```python
from build123d import *

# Parameters (mm, degrees)
EXTRUDE_1_DEPTH              = 5
SKETCH_2_R                   = 6.25
EXTRUDE_2_DEPTH              = 3
SKETCH_3_R                   = 5
EXTRUDE_3_DEPTH              = 5
HOLE_WIZARD_M4_3_D           = 4.5
HOLE_WIZARD_M4_3_CBORE_D     = 8
HOLE_WIZARD_M4_3_CBORE_DEPTH = 4.4
EXTRUDE_4_DEPTH              = 5
EXTRUDE_5_DEPTH              = 5
HOLE_WIZARD_M4_2_D           = 4.5
HOLE_WIZARD_M4_2_CBORE_D     = 8
HOLE_WIZARD_M4_2_CBORE_DEPTH = 4.4
HOLE_WIZARD_M3_1_D           = 3.4
HOLE_WIZARD_M3_1_CBORE_D     = 6.5
HOLE_WIZARD_M3_1_CBORE_DEPTH = 2.5
PATTERN_CIRCULAR_1_COUNT     = 3
PATTERN_CIRCULAR_2_COUNT     = 3
FILLET_2_R                   = 15


with BuildPart() as part:
    # 스케치1 → 보스-돌출1 (new body)
    with BuildSketch(Plane(origin=(0, 0, 0), x_dir=(1, 0, 0), z_dir=(0, 1, 0))):
        with BuildLine():
            Line((-15, 0), (-15, 60))
            ThreePointArc((-15, 60), (0, 75), (15, 60))
            Line((15, 60), (15, 0))
            ThreePointArc((15, 0), (0, -15), (-15, 0))
        make_face()
    extrude(amount=EXTRUDE_1_DEPTH)

    # 스케치2 → 보스-돌출2 (add)
    with BuildSketch(Plane(origin=(0, 5, 0), x_dir=(1, 0, 0), z_dir=(0, 1, 0))):
        with Locations(Location((0, 60, 0), (0, 0, 270))):
            Circle(SKETCH_2_R)
        with Locations(Location((0, 0, 0), (0, 0, 270))):
            Circle(SKETCH_2_R)
    extrude(amount=EXTRUDE_2_DEPTH)

    # 스케치3 → 보스-돌출3 (add)
    with BuildSketch(Plane(origin=(0, 8, 0), x_dir=(1, 0, 0), z_dir=(0, 1, 0))):
        with Locations(Location((0, 60, 0), (0, 0, 270))):
            Circle(SKETCH_3_R)
        with Locations(Location((0, 0, 0), (0, 0, 270))):
            Circle(SKETCH_3_R)
    extrude(amount=EXTRUDE_3_DEPTH)

    # M4 육각 소켓 머리 캡 나사용 카운터보어3 (through all)
    with Locations(Plane(origin=(0, 0, 0), x_dir=(-1, 0, 0), z_dir=(0, -1, 0))):
        with Locations((0, 60), (0, -25)):
            CounterBoreHole(HOLE_WIZARD_M4_3_D / 2, HOLE_WIZARD_M4_3_CBORE_D / 2, HOLE_WIZARD_M4_3_CBORE_DEPTH)

    # 스케치8 → 보스-돌출4 (add)
    with BuildSketch(Plane.XZ):
        with BuildLine():
            Line((-5.13030215, 14.095389312), (23.060476474, 24.355993612))
            ThreePointArc((23.060476474, 24.355993612), (42.286167935, 15.39090645), (33.321080773, -3.834785012))
            Line((33.321080773, -3.834785012), (15, -10.503113073))
            Line((15, -10.503113073), (15, 0))
            ThreePointArc((15, 0), (8.603646545, 12.287280664), (-5.13030215, 14.095389312))
        make_face()
    extrude(amount=-EXTRUDE_4_DEPTH)

    # 스케치9 → 보스-돌출5 (add)
    with BuildSketch(Plane.XZ):
        with BuildLine():
            Line((14.095389312, 5.13030215), (3.834785012, 33.321080773))
            ThreePointArc((3.834785012, 33.321080773), (12.799872174, 52.546772235), (32.025563636, 43.581685073))
            Line((32.025563636, 43.581685073), (42.286167935, 15.39090645))
            ThreePointArc((42.286167935, 15.39090645), (33.321080773, -3.834785012), (14.095389312, 5.13030215))
        make_face()
    extrude(amount=-EXTRUDE_5_DEPTH)

    # M4 육각 소켓 머리 캡 나사용 카운터보어2 (through all)
    with Locations(Plane(origin=(0, 0, 0), x_dir=(-1, 0, 0), z_dir=(0, -1, 0))):
        with Locations((0, 0)):
            CounterBoreHole(HOLE_WIZARD_M4_2_D / 2, HOLE_WIZARD_M4_2_CBORE_D / 2, HOLE_WIZARD_M4_2_CBORE_DEPTH)

    # M3 육각 소켓 머리 캡 나사용 카운터보어1 (through all)
    with Locations(Plane(origin=(0, 0, 0), x_dir=(-1, 0, 0), z_dir=(0, -1, 0))):
        with Locations((-21.008355614, -29.994149336)):
            hole_wizard_m3_1 = CounterBoreHole(HOLE_WIZARD_M3_1_D / 2, HOLE_WIZARD_M3_1_CBORE_D / 2, HOLE_WIZARD_M3_1_CBORE_DEPTH)

    # 원형 패턴1: M3 육각 소켓 머리 캡 나사용 카운터보어1 ×3 about axis
    pattern_circular_1_axis = Axis((17.930174324, 0, 38.451382923), (0, 1, 0))
    for i in range(1, PATTERN_CIRCULAR_1_COUNT):
        add(hole_wizard_m3_1.rotate(pattern_circular_1_axis, i * 360 / PATTERN_CIRCULAR_1_COUNT), mode=Mode.SUBTRACT)

    # 스케치36 → Ø5.0mm 맞춤핀 구멍1 (revolve, cut)
    with BuildSketch(Plane(origin=(14.851993034, 5, 46.90861651), x_dir=(0, 0, 1), z_dir=(1, 0, 0))):
        Polygon((0, 0), (0, 4.002151548), (2.5, 2.5), (2.5, 0), align=None)
    f_5_0mm_1 = revolve(axis=Axis((14.851993034, 11.35, 46.90861651), (0, -1, 0)), mode=Mode.SUBTRACT)

    # 원형 패턴2: Ø5.0mm 맞춤핀 구멍1 ×3 about axis
    pattern_circular_2_axis = Axis((17.930174324, 0, 38.451382923), (0, 1, 0))
    for i in range(1, PATTERN_CIRCULAR_2_COUNT):
        add(f_5_0mm_1.rotate(pattern_circular_2_axis, i * 360 / PATTERN_CIRCULAR_2_COUNT), mode=Mode.SUBTRACT)

    # 필렛2
    fillet_2_edges = [part.edges().sort_by_distance(p)[0] for p in [
        (15, 2.5, -10.503113073),
        (8.965087162, 2.5, 19.225691462),
    ]]
    fillet(fillet_2_edges, radius=FILLET_2_R - 0.0001)  # a hair under: the kernel refuses the full size


solid = part.part
```
Source: CAD feature listing. Evaluate the final solid. Frame: model axes, mm. A direction names the side the tool comes from. Round coordinates to 2 decimals unless told otherwise and drop trailing zeros. Loops run counter-clockwise (first coordinate to the right, second up) from the corner with the lowest first, then second, coordinate; pieces in that order, holes last.
(1) Section query B-B (x = 0). Give the number of separate pieces and of enclosed holes in the cut face, and give its area (3 significant figures).
From the geometry:
separate pieces: 3
enclosed holes: 0
area: 488 mm2
(2) Material intervals for probe 1 along X at (y, z) = (2.25, -60); probe 2 along Z at (x, y) = (0, 3.2); probe 3 along Y at (x, z) = (-4, -49), sorted ascending.
From the geometry:
probe 1: x = -15 to -4, 4 to 15
probe 2: z = -75 to -64, -56 to -4, 4 to 17.25
probe 3: y = 0 to 5
(3) Access query for faces 1 (the flat face through (-2, 4.4, -58)), 2 (the flat face through (5, 8, -58)), 3 (the flat face through (-1, 13, 2.2)). Directions: +Z, -Z, +X, -X, +Y, -Y. A direction counts if a zero-diameter tool reaches every point of the face in a straight line with its end or side. Return the directions, or none.
From the geometry:
face 1: -Y
face 2: +Y
face 3: +Z, -Z, +X, -X, +Y
(4) Pull-direction query (Z, two-part tool) for faces 4 (the cylindrical face through (17.787, 2.535, -12.298)), 5 (the cylindrical face through (41.854, 2.465, 4.071)), 6 (the cylindrical face through (8.85, 3.77, 38.33)); classes: +Z half, -Z half, draft (parallel to the pull), parting line (faces both ways), or undercut.
From the geometry:
face 4: -Z half
face 5: parting line
face 6: undercut
(5) Contact query for flat-ended pins moving along their axis: pin 1 Ø3 at (y, z) = (2.5, 18.5) entering from +X; pin 2 Ø4 at (x, z) = (-0.5, 0.5) entering from -Y; pin 3 Ø4 at (x, z) = (21.01, 29.99) entering from -Y. Output: stop coordinate, or through.
From the geometry:
pin 1: stops at x = 41.7
pin 2: stops at y = 4.4
pin 3: stops at y = 2.5
(6) Section query A-A (y = 11.5). Output: boundary loops of the cut face in (x, z).
From the geometry:
outline: circle Ø10 at (0, -60); circle Ø10 at (0, 0); hole circle Ø4.5 at (0, -60); hole circle Ø4.5 at (0, 0)
(7) Section query C-C (z = 18). Output: boundary loops of the cut face in (x, y), and give its area (3 significant figures).
From the geometry:
outline: (0.75, 0) - (41.34, 0) - (41.34, 5) - (0.75, 5) - close
area: 203 mm2
